```python
from build123d import *
from build123d.topology import SkipClean

# Parameters (mm, degrees)
SKETCH1_R           = 75
BOSS_EXTRUDE1_DEPTH = 15
BOSS_EXTRUDE2_DEPTH = 15
BOSS_EXTRUDE3_START = 15
BOSS_EXTRUDE3_DEPTH = 15


with BuildPart() as part:
    # Sketch1 → Boss-Extrude1 (new body)
    with BuildSketch(Plane(origin=(0, 0, 0), x_dir=(0, 0, -1), z_dir=(1, 0, 0))):
        Circle(SKETCH1_R)
    extrude(amount=BOSS_EXTRUDE1_DEPTH)

    # Sketch2 → Boss-Extrude2 (add)
    with BuildSketch(Plane(origin=(15, 0, 0), x_dir=(0, 0, -1), z_dir=(1, 0, 0))):
        with BuildLine():
            Line((-72.284161474, -20), (72.284161474, -20))
            ThreePointArc((72.284161474, -20), (75, 0), (72.284161474, 20))
            Line((72.284161474, 20), (-72.284161474, 20))
            ThreePointArc((-72.284161474, 20), (-75, 0), (-72.284161474, -20))
        make_face()
    extrude(amount=BOSS_EXTRUDE2_DEPTH)

    # Sketch3 → Boss-Extrude3 (add)
    with SkipClean():  # the faces are left unmerged after this step: merging them gives an invalid solid
        with BuildSketch(Plane.ZY.offset(BOSS_EXTRUDE3_START)):
            with BuildLine():
                Line((-20, 72.284161474), (-20, -72.284161474))
                ThreePointArc((-20, -72.284161474), (0, -75), (20, -72.284161474))
                Line((20, -72.284161474), (20, 72.284161474))
                ThreePointArc((20, 72.284161474), (0, 75), (-20, 72.284161474))
            make_face()
        extrude(amount=-BOSS_EXTRUDE3_DEPTH)


solid = part.part
```
Verification items for the finished model (mm, model axes). A direction names the side the tool comes from. Coordinates: 2 decimals unless noted, no trailing zeros. Loops run counter-clockwise (first coordinate to the right, second up) from the corner with the lowest first, then second, coordinate; pieces in that order, holes last. Notation, with made-up numbers: (13, -12) -> (68, -12) arc R19 ccw to (68, 14) -> close; hole circle Ø3 at (-20, 10.25). An arc over 180 degrees is marked (long way). Put each result on its own line as item: value.
1. Thickness scan on line 1 (X direction, y = -32.5, z = -22); line 2 (X direction, y = -7.5, z = 57.5); line 3 (Z direction, x = -5, y = 41). Record the ranges inside material, lowest first.
Result set:
line 1: x = 0 to 15
line 2: x = 0 to 30
line 3: z = -20 to 20
2. Section check B-B, the plane y = -35.5. Record the boundary of the cut face in (x, z), then the cut area to 3 significant figures.
Result set:
outline: (-15, -20) -> (0, -20) -> (0, -66.07) -> (15, -66.07) -> (15, 66.07) -> (0, 66.07) -> (0, 20) -> (-15, 20) -> close
area: 2,580 mm^2
3. Gauge pin test, flat ends, axial feed: P1, Ø5, axis at y = 0.5, z = 34, coming from the -X side; P2, Ø4.5, axis at x = 25.5, z = -35, coming from the -Y side; P3, Ø8, axis at x = 15, z = 46.5, coming from the +Y side. Record the tip position at first contact, or that the pin passes through.
Result set:
P1: stops at x = 0
P2: stops at y = -20
P3: stops at y = 61.8
4. Tool access check on faces 1 (the face through (-15, 1, 0)), 2 (the face through (15, -41, 1)), 3 (the face through (0, 1, 42)), 4 (the face through (-8, 1, -20)), 5 (the face through (22, 20, -1)). Record the directions out of +Z, -Z, +X, -X, +Y, -Y that give a thin tool (end or side, any length) a straight path to the whole face; none if there is none.
Result set:
face 1: +Z, -Z, -X, +Y, -Y
face 2: +Z, -Z, +X, -Y
face 3: +Z, -X, +Y, -Y
face 4: -Z, -X, +Y, -Y
face 5: +Z, -Z, +X, +Y
5. Section check A-A, the plane x = -4. Record the boundary of the cut face in (y, z).
Result set:
outline: (-72.28, -20) -> (72.28, -20) arc R75 ccw to (72.28, 20) -> (-72.28, 20) arc R75 ccw to start
